Could you check a few things on this drawing? It's one solid part, dimensions in mm from its lowest x, y, z. Give positions to 0.01 mm unless a question says otherwise; leave off trailing zeros. Write each loop counter-clockwise with the first axis right and the second up, starting at its lowest first coordinate (ties: lowest second). Pieces come first, ordered by that corner, then holes.
1. Suppose I cut it at A-A (y = 7). Please give me the cut outline in (x, z), and give its area (3 significant figures).
2. If I drill on probe 1 along Y at (x, z) = (35, 2.55); probe 2 along Y at (x, z) = (5, 0.85); probe 3 along X at (y, z) = (6, 3.4), over which ranges is the centre line in solid material (lowest first)?
3. Suppose I cut it at C-C (y = 75). Please give me the cut outline in (x, z).
4. I'm going to push flat-ended pins straight in: pin 1 (2 mm diameter, centred on y = 38.5, z = 1, fed in from +X); pin 2 (1.2 mm diameter, centred on x = 52.5, z = 1.5, fed in from +Y). Where does each tip first touch, or does it pass through?
5. Suppose I cut it at B-B (z = 3.4). Give the number of separate pieces and of enclosed holes in the cut face, and give its area (3 significant figures).
6. Suppose I cut it at D-D (y = 30). Please give me the cut outline in (x, z).
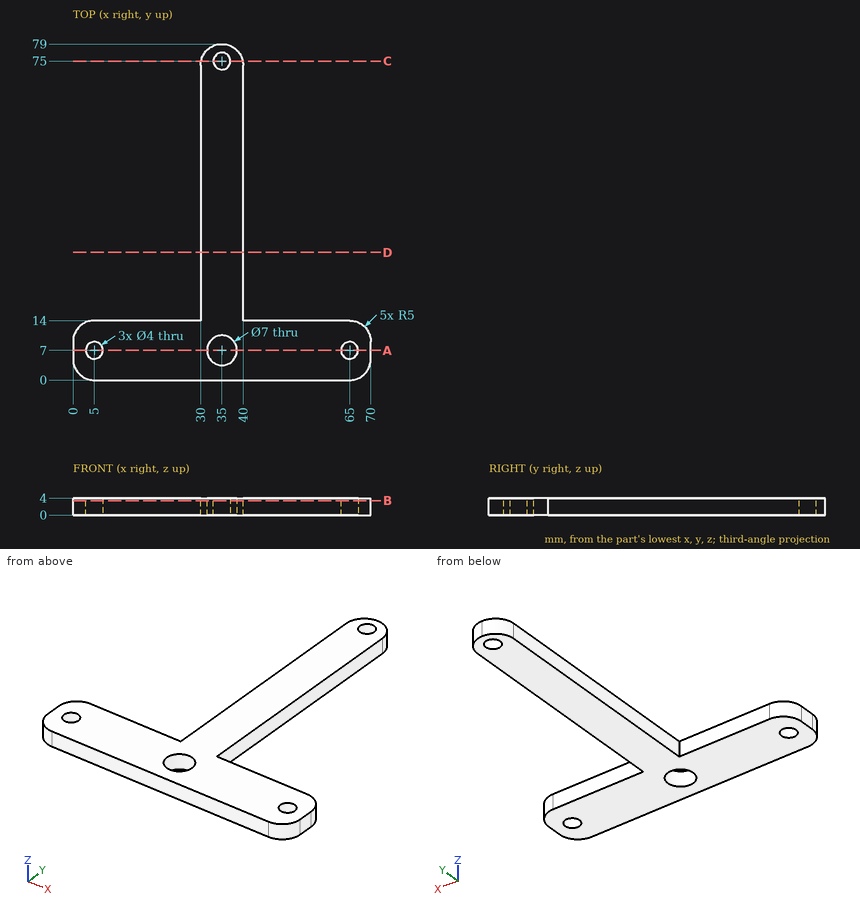
Checks:
1. outline: (0, 0) - (3, 0) - (3, 4) - (0, 4) - close; (7, 0) - (31.5, 0) - (31.5, 4) - (7, 4) - close; (38.5, 0) - (63, 0) - (63, 4) - (38.5, 4) - close; (67, 0) - (70, 0) - (70, 4) - (67, 4) - close
1. area: 220 mm2
2. probe 1: y = 0 to 3.5, 10.5 to 73, 77 to 79
2. probe 2: y = 0 to 5, 9 to 14
2. probe 3: x = 0 to 3.27, 6.73 to 31.65, 38.35 to 63.27, 66.73 to 70
3. outline: (30.1, 0) - (33, 0) - (33, 4) - (30.1, 4) - close; (37, 0) - (39.9, 0) - (39.9, 4) - (37, 4) - close
4. pin 1: stops at x = 40
4. pin 2: stops at y = 14
5. separate pieces: 1
5. enclosed holes: 4
5. area: 1,520 mm2
6. outline: (30, 0) - (40, 0) - (40, 4) - (30, 4) - close
